```python
from build123d import *

# Parameters (mm, degrees)
SALIENTE_EXTRUIR1_DEPTH      = 130
SALIENTE_EXTRUIR1_DEPTH_BACK = 130
REDONDEO1_R                  = 4


with BuildPart() as part:
    # Croquis1 → Saliente-Extruir1 (new, two sides: drawn at the far end of the back side and taken through both)
    with BuildSketch(Plane(origin=(0, 0, 0), x_dir=(0, 0, -1), z_dir=(1, 0, 0)).offset(-SALIENTE_EXTRUIR1_DEPTH_BACK)):
        Polygon((50, 50), (2, 35), (2, 50), (0, 50), (0, 32.279618173), (48, 47.279618173), (48, 0), (48, -47.279618173), (0, -32.279618173), (0, -50), (2, -50), (2, -35), (50, -50), (50, 0), align=None)
    extrude(amount=SALIENTE_EXTRUIR1_DEPTH + SALIENTE_EXTRUIR1_DEPTH_BACK)

    # Redondeo1
    redondeo1_edges = [part.edges().sort_by_distance(p)[0] for p in [
        (0, -50, -50),
        (0, -35, -2),
        (0, -32.279618173, 0),
        (0, -47.279618173, -48),
        (0, 47.279618173, -48),
        (0, 32.279618173, 0),
        (0, 35, -2),
        (0, 50, -50),
    ]]
    fillet(redondeo1_edges, radius=REDONDEO1_R)


solid = part.part
```
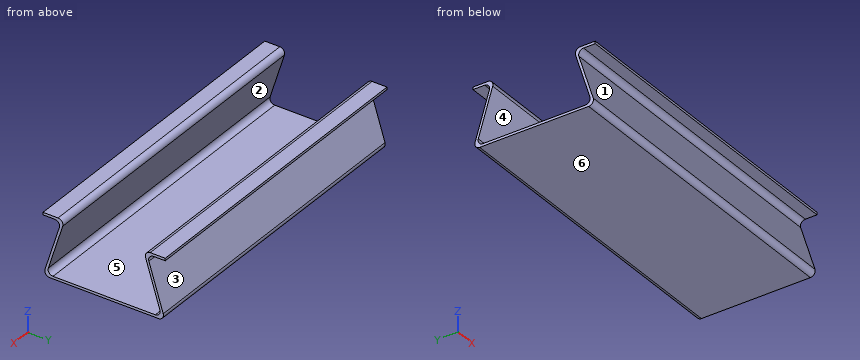
Work out the finished part from the listing and answer in its coordinate system (mm). Face numbers are marked on the shaded views. A direction names the side the tool comes from. Round coordinates to 2 decimals unless told otherwise and drop trailing zeros. Write each loop counter-clockwise with the first axis right and the second up, starting at its lowest first coordinate (ties: lowest second). Pieces come first, ordered by that corner, then holes. Notation, with made-up numbers: (-24, -14) - (15, -14) arc R24 cw to (15, 16) - close; hole circle Ø3 at (-28.75, 12). An arc over 180 degrees is marked (long way). Return JSON: item names as keys, results as strings. Group by question number.
Q1. The part is cut by section C-C on y = -10. Write down the section's boundary in (x, z), then the cut area to 3 significant figures.
Q2. The part is cut by section B-B on x = -91. Write down the section's boundary in (y, z), then the cut area to 3 significant figures.
Q3. Find the intervals of material crossed by L1, parallel to Z at x = -37, y = -25; L2, parallel to Y at x = -99, z = -2.5; L3, parallel to Y at x = -58.5, z = -44 (3 decimals), in increasing order.
Q4. Each of these flat-tipped pins is pushed along its axis until it touches: pin 1 Ø2 at (x, z) = (3.5, -35.5) entering from -Y; pin 2 Ø8 at (x, z) = (52, -16.5) entering from +Y; pin 3 Ø3 at (x, z) = (47.5, -27.5) entering from -Y. Where does it stop, or does it pass through?
Q5. For the marked faces 1 and 2, determine the directions among +Z, -Z, +X, -X, +Y, -Y from which every point of the face is accessible in a straight line to the end or side of a thin tool.
Q6. The part is cut by section A-A on z = -21. Write down the section's boundary in (x, y), then the cut area to 3 significant figures.
Q7. The mould has two halves that part along Y. Classify the marked faces 3, 4, 5 and 6: released by +Y, released by -Y, zero draft, split by the parting line, or undercut.
Solved:
{
 "1": {"outline": "(-130, -50) - (130, -50) - (130, -48) - (-130, -48) - close", "area": "520 mm²"},
 "2": {"outline": "(-50, -2) - (-40.44, -2) arc R4 cw to (-36.62, -7.19) - (-48.38, -44.81) arc R4 ccw to (-44.56, -50) - (44.56, -50) arc R4 ccw to (48.38, -44.81) - (36.62, -7.19) arc R4 cw to (40.44, -2) - (50, -2) - (50, 0) - (37.72, 0) arc R4 ccw to (33.9, -5.19) - (45.66, -42.81) arc R4 cw to (41.84, -48) - (-41.84, -48) arc R4 cw to (-45.66, -42.81) - (-33.9, -5.19) arc R4 ccw to (-37.72, 0) - (-50, 0) - close", "area": "461 mm²"},
 "3": {"L1": "-50 to -48", "L2": "-38.5 to -34.01, 34.01 to 38.5", "L3": "-48.125 to -45.839, 45.839 to 48.125"},
 "4": {"pin 1": "y = -45.78", "pin 2": "y = 40.78", "pin 3": "y = -43.44"},
 "5": {"face 1": "+X, -X, -Y", "face 2": "+X, -X"},
 "6": {"outline": "(-130, -40.94) - (130, -40.94) - (130, -38.84) - (-130, -38.84) - close; (-130, 38.84) - (130, 38.84) - (130, 40.94) - (-130, 40.94) - close", "area": "1,090 mm²"},
 "7": {"face 3": "released by +Y", "face 4": "undercut", "face 5": "undercut", "face 6": "zero draft"}
}
